```python
from build123d import *

# Parameters (mm, degrees)
BOSS_EXTRUDE1_DEPTH     = 10
SKETCH2_R               = 1.5
CUT_EXTRUDE1_DEPTH      = 1
CUT_EXTRUDE1_DEPTH_BACK = 9
CHAMFER1_SIZE           = 0.2
SKETCH4_R               = 1.5
BOSS_EXTRUDE2_DEPTH     = 6.5
CHAMFER2_SIZE           = 0.6


with BuildPart() as part:
    # Sketch1 → Boss-Extrude1 (new body)
    with BuildSketch(Plane.XY):
        Polygon((2.621170222, 0), (1.310585111, 2.27), (-1.310585111, 2.27), (-2.621170222, 0), (-1.310585111, -2.27), (1.310585111, -2.27), align=None)
    extrude(amount=BOSS_EXTRUDE1_DEPTH)

    # Sketch2 → Cut-Extrude1 (cut, two sides)
    with BuildSketch(Plane.XY.offset(10)) as cut_extrude1_sk:
        Circle(SKETCH2_R)
    extrude(amount=CUT_EXTRUDE1_DEPTH, mode=Mode.SUBTRACT)
    extrude(cut_extrude1_sk.sketch, amount=-CUT_EXTRUDE1_DEPTH_BACK, mode=Mode.SUBTRACT)

    # Sketch3 → Cut-Revolve1 (revolve, cut)
    with BuildSketch(Plane(origin=(0, 0, 0), x_dir=(1, 0, 0), z_dir=(0, 1, 0))):
        Polygon((-2.621170222, -10), (-2.271170222, -10), (-2.621170222, -9.8), align=None)
    revolve(axis=Axis((0, 0, 1), (0, 0, 1)), mode=Mode.SUBTRACT)

    # Chamfer1
    chamfer1_edges = [part.edges().sort_by_distance(p)[0] for p in [
        (-1.5, 0, 10),
    ]]
    chamfer(chamfer1_edges, length=CHAMFER1_SIZE)

    # Sketch4 → Boss-Extrude2 (add)
    with BuildSketch(Plane(origin=(0, 0, 0), x_dir=(-1, 0, 0), z_dir=(0, 0, -1))):
        Circle(SKETCH4_R)
    extrude(amount=BOSS_EXTRUDE2_DEPTH)

    # Chamfer2
    chamfer2_edges = [part.edges().sort_by_distance(p)[0] for p in [
        (1.5, 0, -6.5),
    ]]
    chamfer(chamfer2_edges, length=CHAMFER2_SIZE)


solid = part.part
```
Design review of the part built by this model. Coordinates are the model's own, in mm. A direction names the side the tool comes from. Coordinates: 2 decimals unless noted, no trailing zeros. Order: outer loops, then holes, each group sorted by start corner. A loop starts at its lowest first (then second) coordinate and runs counter-clockwise, first axis right, second up.
1) For faces 4 (the cylindrical face through (-1.5, 0.07, 5.46)), 5 (the flat face through (0, 0, -6.5)), 6 (the cylindrical face through (1.5, 0.07, -2.91)), list the 3-axis set-ups (+Z, -Z, +X, -X, +Y, -Y) from which the entire face can be reached by the end or side of a thin tool; tool diameter is ignored.
2) Take a section at A-A, the plane z = 8.5. Give the boundary of the cut face in (x, y).
3) Wall thickness on line 1 along Y through (x, z) = (0, 5.5); line 2 along Y through (x, z) = (1.2, 4.5); line 3 along Y through (x, z) = (2, 2.75): over which ranges is each line inside the solid? List them lowest first.
4) Mouldability with a two-part tool opening along Y and no side actions: class faces 1 (the flat face through (-2, 0, 10)), 2 (the flat face through (0, 0, 1)), 3 (the flat face through (-1.957, 1.151, 4.93)) as +Y half, -Y half, draft (parallel to the pull), parting line (faces both ways), or undercut.
5) Take a section at B-B, the plane z = -0.5. Give the boundary of the cut face in (x, y), and give its area (3 significant figures).
6) Clearance check with flat-ended pins moving along their axes: pin 1 (2 mm diameter, centred on x = 2, y = -1, fed in from -Z); pin 2 (2 mm diameter, centred on y = -2, z = 3.5, fed in from +X); pin 3 (2 mm diameter, centred on x = -1.5, z = -2.5, fed in from -Y). State where each tip first meets the part, or that it passes through.
Returned:
1. face 4: +Z
1. face 5: -Z, +X, -X, +Y, -Y
1. face 6: -Z
2. outline: (-2.62, 0) - (-1.31, -2.27) - (1.31, -2.27) - (2.62, 0) - (1.31, 2.27) - (-1.31, 2.27) - close; hole circle Ø3 at (0, 0)
3. line 1: y = -2.27 to -1.5, 1.5 to 2.27
3. line 2: y = -2.27 to -0.9, 0.9 to 2.27
3. line 3: y = -1.08 to 1.08
4. face 1: draft
4. face 2: undercut
4. face 3: +Y half
5. outline: circle Ø3 at (0, 0)
5. area: 7.07 mm2
6. pin 1: stops at z = -6.16
6. pin 2: stops at x = 2.04
6. pin 3: stops at y = -1.41
